Part print with two shaded views. Sizes in mm from the minimum x, y, z corner. Give positions to 0.01 mm unless a question says otherwise; leave off trailing zeros. Order: outer loops, then holes, each group sorted by start corner. A loop starts at its lowest first (then second) coordinate and runs counter-clockwise, first axis right, second up. Notation, with made-up numbers: M 1.5,-36.75 L 15.5,-36.75 A36 cw 15.5,0.25 Z; hole C 43,-2 d9. An arc over 180 degrees is marked long. Return JSON: item names as keys, results as strings.
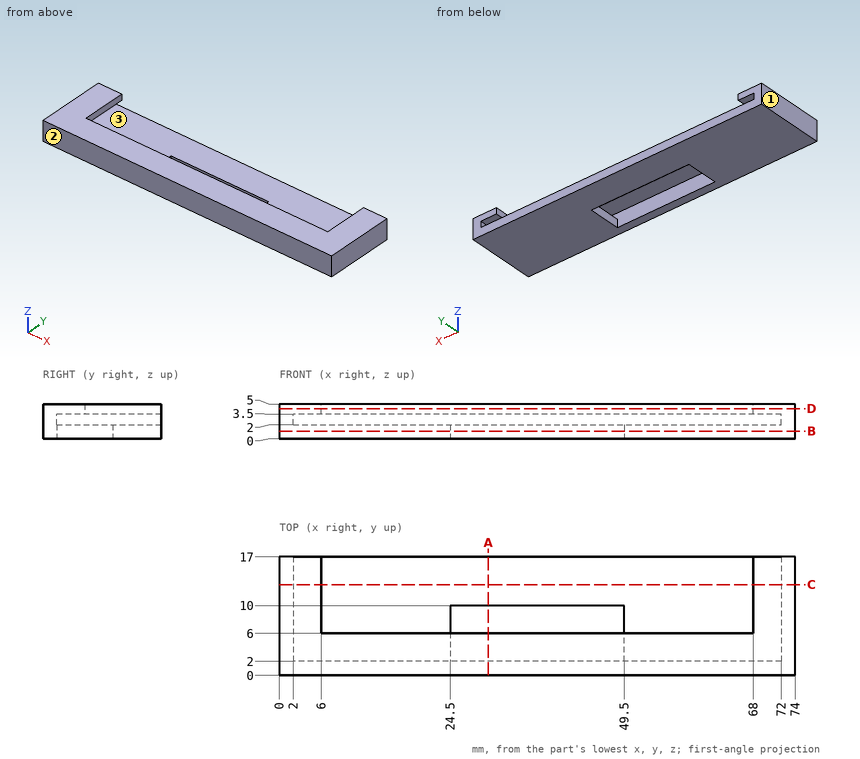
Q1. Band-saw the part on D-D (z = 4.35). Give the cut face in (x, y).
Established:
{"outline": "M 0,0 L 74,0 L 74,17 L 68,17 L 68,6 L 6,6 L 6,17 L 0,17 Z"}
Q2. Band-saw the part on C-C (y = 13). Give the cut face in (x, z).
Established:
{"outline": "M 0,0 L 74,0 L 74,5 L 68,5 L 68,3.5 L 72,3.5 L 72,2 L 2,2 L 2,3.5 L 6,3.5 L 6,5 L 0,5 Z"}
Q3. Band-saw the part on B-B (z = 1.1). Give the cut face in (x, y).
Established:
{"outline": "M 0,0 L 74,0 L 74,17 L 0,17 Z; hole M 24.5,2 L 49.5,2 L 49.5,10 L 24.5,10 Z"}
Q4. Two-plate mould, pull along X, no slides. Class the marked faces 1, 2 and 3: +X half, -X half, draft (parallel to the pull), parting line (faces both ways), or undercut.
Established:
{"face 1": "-X half", "face 2": "draft", "face 3": "undercut"}
Q5. Probe line 1 along X through (y, z) = (6.75, 2.5); line 2 along Z through (x, y) = (19, 5.5); line 3 along X through (y, z) = (4.5, 1.7). List the from-to ranges inside material, lowest first.
Established:
{"line 1": "x = 0 to 2, 72 to 74", "line 2": "z = 0 to 2, 3.5 to 5", "line 3": "x = 0 to 24.5, 49.5 to 74"}
Q6. Band-saw the part on A-A (x = 30). Give the cut face in (y, z).
Established:
{"outline": "M 0,0 L 2,0 L 2,3.5 L 6,3.5 L 6,5 L 0,5 Z; M 10,0 L 17,0 L 17,2 L 10,2 Z"}
Q7. Pin check, flat tip, straight feed: pin 1 (0.8 mm diameter, centred on x = 41, z = 4, fed in from +Y). Stop position of the tip, or through.
Established:
{"pin 1": "stops at y = 6"}
